Build history of the part. All positions in model axes, mm. Face numbers are marked on the shaded views. A direction names the side the tool comes from. Round coordinates to 2 decimals unless told otherwise and drop trailing zeros. Write each loop counter-clockwise with the first axis right and the second up, starting at its lowest first coordinate (ties: lowest second). Pieces come first, ordered by that corner, then holes. Notation, with made-up numbers: (-2, -11) -> (21, -11) arc R14 cw to (21, 0) -> close; hole circle Ø11 at (-25, 75.5). An arc over 180 degrees is marked (long way). Answer in a Markdown table with one row per item.
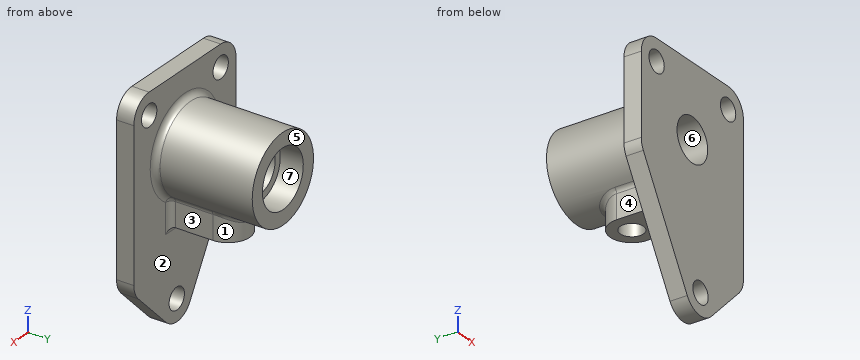
Autodesk Inventor part; units mm, degrees
ref_plane "YZ Plane" through (0, 0, 0) normal (1, 0, 0) x (0, 1, 0)
ref_plane "XZ Plane" through (0, 0, 0) normal (0, 1, 0) x (-1, 0, 0)
ref_plane "XY Plane" through (0, 0, 0) normal (0, 0, 1) x (1, 0, 0)
sketch "Sketch1" plane through (0, 0, 0) normal (0, 1, 0) x (-1, 0, 0)
  line L0 (35, 50) -> (-35, 50)
  line L1 (-50, 35) -> (-50, -68)
  line L2 (-45.6066, -78.6066) -> (-18.6066, -105.6066)
  line L3 (4.9904, -102.5) -> (47.9904, -28.0218)
  line L4 (50, -20.5218) -> (50, 35)
  line L5 (0, -144.3313) -> (0, 86.0129) construction
  arc A0 (-18.6066, -105.6066) -> (4.9904, -102.5) centre (-8, -95) ccw
  arc A1 (47.9904, -28.0218) -> (50, -20.5218) centre (35, -20.5218) ccw
  arc A2 (50, 35) -> (35, 50) centre (35, 35) ccw
  arc A3 (-35, 50) -> (-50, 35) centre (-35, 35) ccw
  arc A4 (-50, -68) -> (-45.6066, -78.6066) centre (-35, -68) ccw
  point P0 (0, 0)
  point P1 (50, 50)
  point P2 (-50, 50)
  point P3 (0, 50)
  dimension "d0" = 100
  dimension "d1" = 50
  dimension "d2" = 135
  dimension "d3" = 15
  dimension "d4" = 42
  dimension "d5" = 145
  dimension "d6" = 30
  dimension "d7" = 15
extrude "Extrusion1" add sketch "Sketch1" along normal blind 12
sketch "Sketch2" plane through (0, 12, 0) normal (0, 1, 0) x (1, 0, 0)
  arc A0 (35, -50) -> (50, -35) centre (35, -35) ccw
  arc A1 (-50, -35) -> (-35, -50) centre (-35, -35) ccw
  arc A2 (18.6066, 105.6066) -> (-4.9904, 102.5) centre (8, 95) ccw
  point P0 (0, 0)
hole "Hole1" at (35, 12, 35) at (-35, 12, 35) at (8, 12, -95) direction (0, -1, 0) diameter 15 end through all
sketch "Sketch3" plane through (0, 12, 0) normal (0, 1, 0) x (1, 0, 0)
  circle A0 centre (0, 0) radius 30
  dimension "d17" = 60
extrude "Extrusion2" add sketch "Sketch3" along normal blind 68
sketch "Sketch5" plane through (0, 0, 0) normal (0, 0, 1) x (1, 0, 0)
  arc A0 (15, 42) -> (-15, 42) centre (0, 42) ccw
  line L0 (15, 42) -> (15, 0)
  line L1 (-15, 42) -> (-15, 0)
  line L2 (15, 0) -> (-15, 0)
  line L3 (-70, 0) -> (70, 0) construction
  point P0 (0, 0)
  dimension "d39" = 30
  dimension "d41" = 42
extrude "Extrusion4" add sketch "Sketch5" against normal blind 45
sketch "Sketch6" plane through (0, 80, 0) normal (0, 1, 0) x (1, 0, 0)
  circle A0 centre (0, 0) radius 30
hole "Hole3" at (0, 80, 0) direction (0, -1, 0) diameter 30 end through all counterbore diameter 40 counterbore depth 16
sketch "Sketch7" plane through (0, 0, -45) normal (0, 0, -1) x (-1, 0, 0)
  arc A0 (15, 42) -> (-15, 42) centre (0, 42) ccw
  point P0 (0, 0)
hole "Hole4" at (0, 42, -45) direction (0, 0, 1) diameter 16 end up to surface
fillet "Fillet1" radius 4 7 edges at (25.9808, 12, -15) (-15, 12, 25.9808) (15, 12, -35.4904) (-15, 27, -25.9808) (15, 27, -25.9808) (-0.0148, 57, -30) (0, 12, -45)
properties material "Steel, Carbon"
Q1. Saw through at C-C on z = 38.5. Write the cut outline in (x, y).
A:
| item | result |
|---|---|
| outline | (-49.59, 0) -> (-41.63, 0) -> (-41.63, 12) -> (-49.59, 12) -> close; (-28.37, 0) -> (28.37, 0) -> (28.37, 12) -> (-28.37, 12) -> close; (41.63, 0) -> (49.59, 0) -> (49.59, 12) -> (41.63, 12) -> close |
Q2. Wall check: line 1 (X direction, y = 5, z = 35); line 2 (Z direction, x = 0, y = 19); line 3 (X direction, y = 73, z = 0). Give the ranges that are in metal, low to high. Write a range as [from, to].
A:
| item | result |
|---|---|
| line 1 | [-50, -42.5], [-27.5, 27.5], [42.5, 50] |
| line 2 | [-45, -15], [15, 30] |
| line 3 | [-30, -20], [20, 30] |
Q3. Drop flat-ended pins along their axis: P1, Ø16.5, axis at y = 25, z = -37, coming from the -X side; P2, Ø1.5, axis at x = -31.5, z = -40.5, coming from the +Y side; P3, Ø1.5, axis at x = 10, y = 32, coming from the +Z side; P4, Ø24, axis at x = 0, z = 0, coming from the +Y side. Give the stop position or say it passes through.
A:
| item | result |
|---|---|
| P1 | x = -15 |
| P2 | y = 12 |
| P3 | z = 28.54 |
| P4 | through |
Q4. Saw through at B-B on y = 22.5. Write the cut outline in (x, z).
A:
| item | result |
|---|---|
| outline | (-16.76, -24.88) arc R4 cw to (-15, -28.2) -> (-15, -45) -> (15, -45) -> (15, -28.2) arc R4 cw to (16.76, -24.88) arc R30 ccw (long way) to start; hole circle Ø30 at (0, 0) |
Q5. Two-plate mould, pull along X, no slides. Class the marked faces 4, 5, 6 and 7: released by +X, released by -X, zero draft, split by the parting line, or undercut.
A:
| item | result |
|---|---|
| face 4 | released by -X |
| face 5 | zero draft |
| face 6 | undercut |
| face 7 | undercut |
Q6. Saw through at A-A on z = 0. Write the cut outline in (x, y).
A:
| item | result |
|---|---|
| outline | (-50, 0) -> (-15, 0) -> (-15, 64) -> (-20, 64) -> (-20, 80) -> (-30, 80) -> (-30, 16) arc R4 cw to (-34, 12) -> (-50, 12) -> close; (15, 0) -> (50, 0) -> (50, 12) -> (34, 12) arc R4 cw to (30, 16) -> (30, 80) -> (20, 80) -> (20, 64) -> (15, 64) -> close |
Q7. Saw through at D-D on z = -95. Write the cut outline in (x, y), plus the area to 3 significant figures.
A:
| item | result |
|---|---|
| outline | (-9.32, 0) -> (0.5, 0) -> (0.5, 12) -> (-9.32, 12) -> close; (15.5, 0) -> (29.21, 0) -> (29.21, 12) -> (15.5, 12) -> close |
| area | 282 mm² |
Q8. Which spindle directions (+Z, -Z, +X, -X, +Y, -Y) get a long thin tool onto all of the face, cutting with end or side? Do the marked faces 1, 2 and 3. Say none if no direction does.
A:
| item | result |
|---|---|
| face 1 | -Z, +Y |
| face 2 | +Y |
| face 3 | -Z, +X, +Y |
